Design review of the part built by this model. Coordinates are the model's own, in mm. A direction names the side the tool comes from. Coordinates: 2 decimals unless noted, no trailing zeros. Loops run counter-clockwise (first coordinate to the right, second up) from the corner with the lowest first, then second, coordinate; pieces in that order, holes last. Notation, with made-up numbers: M 37,88.5 L 72,88.5 A11 cw 72,97.5 Z; hole C 62,-12 d3. An arc over 180 degrees is marked long. One line per item, written item: value.
```python
from build123d import *

# Parameters (mm, degrees)
BOSS_EXTRUDE1_DEPTH              = 10
BOSS_EXTRUDE2_DEPTH              = 30
BOSS_EXTRUDE3_DEPTH              = 10
M8_CLEARANCE_HOLE1_D             = 9
TAP_DRILL_FOR_M8X1_25_TAP1_D     = 6.8
TAP_DRILL_FOR_M8X1_25_TAP1_DEPTH = 15
TAP_DRILL_FOR_M8X1_25_TAP1_TIP   = 2.042926105
M6_CLEARANCE_HOLE1_D             = 6.6


with BuildPart() as part:
    # Sketch1 → Boss-Extrude1 (new body)
    with BuildSketch(Plane.XY):
        with BuildLine():
            Line((2, 0), (58, 0))
            ThreePointArc((58, 0), (59.414213562, 0.585786438), (60, 2))
            Line((60, 2), (60, 13))
            ThreePointArc((60, 13), (59.414213562, 14.414213562), (58, 15))
            Line((58, 15), (19.5, 15))
            ThreePointArc((19.5, 15), (18.085786438, 15.585786438), (17.5, 17))
            Line((17.5, 17), (17.5, 23.75))
            ThreePointArc((17.5, 23.75), (8.75, 32.5), (0, 23.75))
            Line((0, 23.75), (0, 2))
            ThreePointArc((0, 2), (0.585786438, 0.585786438), (2, 0))
        make_face()
    boss_extrude1 = extrude(amount=-BOSS_EXTRUDE1_DEPTH)

    # Sketch2 → Boss-Extrude2 (add)
    with BuildSketch(Plane(origin=(0, 0, -10), x_dir=(-1, 0, 0), z_dir=(0, 0, -1))):
        with BuildLine():
            Line((-58, 0), (-2, 0))
            ThreePointArc((-2, 0), (-0.585786438, 0.585786438), (0, 2))
            Line((0, 2), (0, 15))
            Line((0, 15), (-58, 15))
            ThreePointArc((-58, 15), (-59.414213562, 14.414213562), (-60, 13))
            Line((-60, 13), (-60, 2))
            ThreePointArc((-60, 2), (-59.414213562, 0.585786438), (-58, 0))
        make_face()
    boss_extrude2 = extrude(amount=BOSS_EXTRUDE2_DEPTH)

    # Mirror2: Boss-Extrude2 across plane
    add(boss_extrude2.mirror(Plane(origin=(0, 0, -40), x_dir=(1, 0, 0), z_dir=(0, 0, -1))))

    # Mirror3: Boss-Extrude1 across plane
    add(boss_extrude1.mirror(Plane(origin=(0, 0, -40), x_dir=(1, 0, 0), z_dir=(0, 0, -1))))

    # Sketch3 → Boss-Extrude3 (add, symmetric)
    with BuildSketch(Plane(origin=(0, 0, -40), x_dir=(-1, 0, 0), z_dir=(0, 0, -1))):
        with BuildLine():
            Line((-57, 15), (-40, 15))
            ThreePointArc((-40, 15), (-43.192782494, 25.890045982), (-50.202268973, 34.814958355))
            ThreePointArc((-50.202268973, 34.814958355), (-51.150466942, 35.015879251), (-51.823619098, 34.318516526))
            Line((-51.823619098, 34.318516526), (-57, 15))
        make_face()
    extrude(amount=BOSS_EXTRUDE3_DEPTH, both=True)

    # M8 Clearance Hole1 (through all)
    with Locations(Plane.XY):
        with Locations((8.75, 23.75)):
            Hole(M8_CLEARANCE_HOLE1_D / 2)

    # Tap Drill for M8x1.25 Tap1
    with Locations(Plane(origin=(-0.592221329, 33.928337229, 0), x_dir=(0, 0, 1), z_dir=(-0.017452406437290298, 0.9998476951563912, 0))):
        with Locations((-40, 46.802227727)):
            Hole(TAP_DRILL_FOR_M8X1_25_TAP1_D / 2, depth=TAP_DRILL_FOR_M8X1_25_TAP1_DEPTH)
            with Locations((0, 0, -(TAP_DRILL_FOR_M8X1_25_TAP1_DEPTH + TAP_DRILL_FOR_M8X1_25_TAP1_TIP / 2))):  # 118° drill point
                Cone(0, TAP_DRILL_FOR_M8X1_25_TAP1_D / 2, TAP_DRILL_FOR_M8X1_25_TAP1_TIP, mode=Mode.SUBTRACT)

    # M6 Clearance Hole1 (through all)
    with Locations(Plane(origin=(0, 15, 0), x_dir=(1, 0, 0), z_dir=(0, 1, 0))):
        with Locations((38, 15), (38, 65)):
            Hole(M6_CLEARANCE_HOLE1_D / 2)


solid = part.part
```
(1) Tool access review of faces 1 (the cylindrical face through (8.9, 32.5, -4.9)), 2 (the flat face through (49, 23, -50)), 3 (the cylindrical face through (49.74, 25.34, -39.56)), 4 (the flat face through (12, 20, -70)): name each direction out of +Z, -Z, +X, -X, +Y, -Y from which nothing blocks a thin tool from reaching the whole face with its end or side.
Reply:
face 1: +Z, -Z, +Y
face 2: -Z, +X, -X, +Y
face 3: none
face 4: +X, -X, +Y
(2) Mouldability with a two-part tool opening along X and no side actions: class faces 5 (the flat face through (23, 9, 0)), 6 (the cylindrical face through (6.331, 27.544, -5.07)), 7 (the flat face through (17.5, 20, -5)) as released by +X, released by -X, zero draft, split by the parting line, or undercut.
Reply:
face 5: zero draft
face 6: undercut
face 7: released by +X
(3) We need section A-A on z = -65. State the section outline as (x, y) points, then the cut area to 3 significant figures.
Reply:
outline: M 0,2 A2 ccw 2,0 L 34.7,0 L 34.7,15 L 0,15 Z; M 41.3,0 L 58,0 A2 ccw 60,2 L 60,13 A2 ccw 58,15 L 41.3,15 Z
area: 798 mm2
(4) We need section B-B on x = 8.75. State the section outline as (y, z) points, then the cut area to 3 significant figures.
Reply:
outline: M 0,-80 L 19.25,-80 L 19.25,-70 L 15,-70 L 15,-10 L 19.25,-10 L 19.25,0 L 0,0 Z; M 28.25,-80 L 32.5,-80 L 32.5,-70 L 28.25,-70 Z; M 28.25,-10 L 32.5,-10 L 32.5,0 L 28.25,0 Z
area: 1,370 mm2
(5) We need section D-D on x = 38. State the section outline as (y, z) points, then the cut area to 3 significant figures.
Reply:
outline: M 0,-80 L 15,-80 L 15,-68.3 L 0,-68.3 Z; M 0,-61.7 L 15,-61.7 L 15,-18.3 L 0,-18.3 Z; M 0,-11.7 L 15,-11.7 L 15,0 L 0,0 Z
area: 1,000 mm2
(6) Insertion check: pin 1 (8.5 mm diameter, centred on x = 51, y = 25.5, fed in from +Z); pin 2 (5 mm diameter, centred on x = 23, z = -23.5, fed in from +Y); pin 3 (8 mm diameter, centred on x = 36, z = -44, fed in from -Y); pin 4 (2 mm diameter, centred on y = 19.5, z = -5.5, fed in from +X). Each pin has a flat end and moves straight along its axis. Give the tip position at first contact, or say it passes through.
Reply:
pin 1: stops at z = -30
pin 2: stops at y = 15
pin 3: stops at y = 0
pin 4: stops at x = 17.5
(7) We need section C-C on z = -27. State the section outline as (x, y) points.
Reply:
outline: M 0,2 A2 ccw 2,0 L 58,0 A2 ccw 60,2 L 60,13 A2 ccw 58,15 L 0,15 Z
(8) To check wall thickness, follow line 1 along Z through (x, y) = (38, 10.75); line 2 along X through (y, z) = (9, -15); line 3 along Y through (x, z) = (8.75, -74). State the ranges of each line that lie inside material, in increasing order. Write a range as [from, to].
Reply:
line 1: z = [-80, -68.3], [-61.7, -18.3], [-11.7, 0]
line 2: x = [0, 34.7], [41.3, 60]
line 3: y = [0, 19.25], [28.25, 32.5]
